Geometry: see drawing. Coordinates: mm, zero at the bounding-box minimum. Coordinates: 2 decimals unless noted, no trailing zeros. Order: outer loops, then holes, each group sorted by start corner. A loop starts at its lowest first (then second) coordinate and runs counter-clockwise, first axis right, second up.
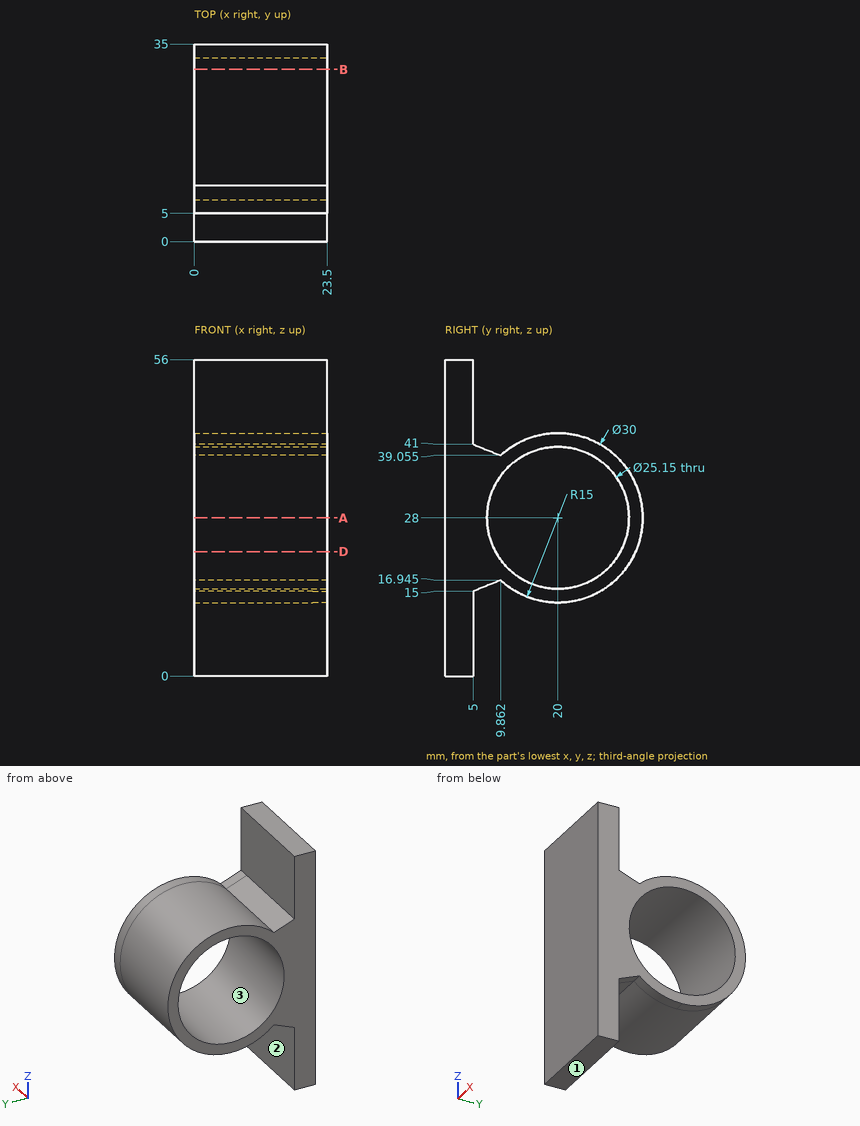
Q1. Material intervals for line 1 along Y through (x, z) = (10, 28) (1 decimal); line 2 along Z through (x, y) = (14.5, 20) (1 decimal); line 3 along Y through (x, z) = (13, 17) (1 decimal), sorted ascending.
Solutions:
line 1: y = 0 to 7.4, 32.6 to 35
line 2: z = 13 to 15.4, 40.6 to 43
line 3: y = 0 to 13.9, 26.1 to 30.2
Q2. Section query D-D on z = 22. Output: boundary loops of the cut face in (x, y).
Solutions:
outline: (0, 0) - (23.5, 0) - (23.5, 8.95) - (0, 8.95) - close; (0, 31.05) - (23.5, 31.05) - (23.5, 33.75) - (0, 33.75) - close
Q3. Section query B-B on y = 30.5. Output: boundary loops of the cut face in (x, z), plus the area to 3 significant figures.
Solutions:
outline: (0, 17.29) - (23.5, 17.29) - (23.5, 21.08) - (0, 21.08) - close; (0, 34.92) - (23.5, 34.92) - (23.5, 38.71) - (0, 38.71) - close
area: 178 mm2
Q4. Section query A-A on z = 28. Output: boundary loops of the cut face in (x, y) (1 decimal).
Solutions:
outline: (0, 0) - (23.5, 0) - (23.5, 7.4) - (0, 7.4) - close; (0, 32.6) - (23.5, 32.6) - (23.5, 35) - (0, 35) - close
Q5. Pin query (flat end, axial travel): P1, Ø12, axis at x = 8.5, z = 47.5, coming from the +Y side; P2, Ø12, axis at x = 7.5, z = 41.5, coming from the +Y side; P3, Ø1, axis at x = 4.5, y = 12, coming from the -Z side. Return the tip coordinate at first contact, or that it passes through.
Solutions:
P1: stops at y = 26.54
P2: stops at y = 32.99
P3: stops at z = 15.01
Q6. Pull-direction query (Z, two-part tool) for the marked faces 1, 2 and 3; classes: pulls with the +Z half, pulls with the -Z half, needs draft (parallel to the pull), parting line crosses it, or undercut.
Solutions:
face 1: pulls with the -Z half
face 2: needs draft
face 3: undercut
